Verification items for the finished model (mm, model axes). Give positions to 0.01 mm unless a question says otherwise; leave off trailing zeros. Write each loop counter-clockwise with the first axis right and the second up, starting at its lowest first coordinate (ties: lowest second). Pieces come first, ordered by that corner, then holes. Notation, with made-up numbers: (-1, -10.5) -> (53, -10.5) arc R24 cw to (53, 19.5) -> close; hole circle Ø11 at (-31, 57.5). An arc over 180 degrees is marked (long way). Write item = value, one per line.
from build123d import *

# Parameters (mm, degrees)
SKETCH1_W           = 127
SKETCH1_H           = 76.2
BOSS_EXTRUDE1_DEPTH = 6.35
CUT_EXTRUDE1_REACH  = 8.35
SKETCH2_R           = 1.905


with BuildPart() as part:
    # Sketch1 → Boss-Extrude1 (new body)
    with BuildSketch(Plane.XY):
        with Locations((63.5, -38.1)):
            Rectangle(SKETCH1_W, SKETCH1_H)
    extrude(amount=BOSS_EXTRUDE1_DEPTH)

    # Sketch2 → Cut-Extrude1 (cut, up to next)
    with BuildSketch(Plane.XY.offset(6.35), mode=Mode.PRIVATE) as cut_extrude1_sk1:
        with Locations((82.55, -31.75)):
            Circle(SKETCH2_R)
    cut_extrude1_tool1 = extrude(cut_extrude1_sk1.sketch, amount=-CUT_EXTRUDE1_REACH, mode=Mode.PRIVATE) & part.part
    add(cut_extrude1_tool1.solids().sort_by_distance((82.55, -31.75, 6.35))[0], mode=Mode.SUBTRACT)
    # Sketch2 → Cut-Extrude1 (cut, up to next)
    with BuildSketch(Plane.XY.offset(6.35), mode=Mode.PRIVATE) as cut_extrude1_sk2:
        with Locations((120.65, -31.75)):
            Circle(SKETCH2_R)
    cut_extrude1_tool2 = extrude(cut_extrude1_sk2.sketch, amount=-CUT_EXTRUDE1_REACH, mode=Mode.PRIVATE) & part.part
    add(cut_extrude1_tool2.solids().sort_by_distance((120.65, -31.75, 6.35))[0], mode=Mode.SUBTRACT)
    # Sketch2 → Cut-Extrude1 (cut, up to next)
    with BuildSketch(Plane.XY.offset(6.35), mode=Mode.PRIVATE) as cut_extrude1_sk3:
        with Locations((82.55, -69.85)):
            Circle(SKETCH2_R)
    cut_extrude1_tool3 = extrude(cut_extrude1_sk3.sketch, amount=-CUT_EXTRUDE1_REACH, mode=Mode.PRIVATE) & part.part
    add(cut_extrude1_tool3.solids().sort_by_distance((82.55, -69.85, 6.35))[0], mode=Mode.SUBTRACT)
    # Sketch2 → Cut-Extrude1 (cut, up to next)
    with BuildSketch(Plane.XY.offset(6.35), mode=Mode.PRIVATE) as cut_extrude1_sk4:
        with Locations((120.65, -69.85)):
            Circle(SKETCH2_R)
    cut_extrude1_tool4 = extrude(cut_extrude1_sk4.sketch, amount=-CUT_EXTRUDE1_REACH, mode=Mode.PRIVATE) & part.part
    add(cut_extrude1_tool4.solids().sort_by_distance((120.65, -69.85, 6.35))[0], mode=Mode.SUBTRACT)
    # Sketch2 → Cut-Extrude1 (cut, up to next)
    with BuildSketch(Plane.XY.offset(6.35), mode=Mode.PRIVATE) as cut_extrude1_sk5:
        with Locations((6.35, -50.8)):
            Circle(SKETCH2_R)
    cut_extrude1_tool5 = extrude(cut_extrude1_sk5.sketch, amount=-CUT_EXTRUDE1_REACH, mode=Mode.PRIVATE) & part.part
    add(cut_extrude1_tool5.solids().sort_by_distance((6.35, -50.8, 6.35))[0], mode=Mode.SUBTRACT)


solid = part.part
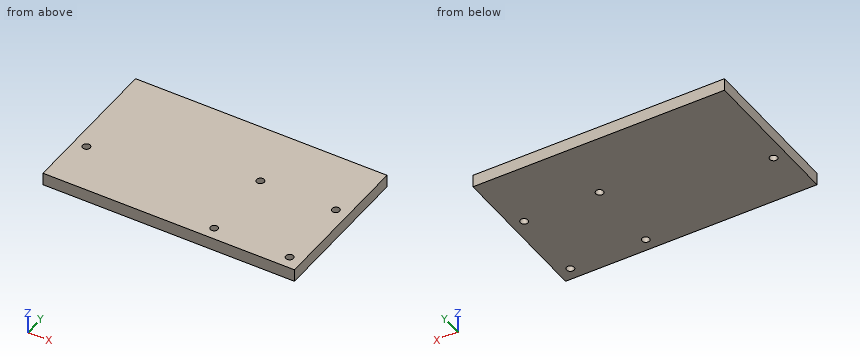
Item 1: Sectioned sample at C-C on y = -31.75. Record the cut outline in (x, z) (3 decimals), then the cut area to 3 significant figures.
Response values:
outline = (0, 0) -> (80.645, 0) -> (80.645, 6.35) -> (0, 6.35) -> close; (84.455, 0) -> (118.745, 0) -> (118.745, 6.35) -> (84.455, 6.35) -> close; (122.555, 0) -> (127, 0) -> (127, 6.35) -> (122.555, 6.35) -> close
area = 758 mm^2
Item 2: Sectioned sample at A-A on y = -50.8. Record the cut outline in (x, z) (3 decimals), then the cut area to 3 significant figures.
Response values:
outline = (0, 0) -> (4.445, 0) -> (4.445, 6.35) -> (0, 6.35) -> close; (8.255, 0) -> (127, 0) -> (127, 6.35) -> (8.255, 6.35) -> close
area = 782 mm^2
Item 3: Material ranges on line 1 (X direction, y = -69.85, z = 1.75) (3 decimals); line 2 (Y direction, x = 82.55, z = 2.25) (3 decimals); line 3 (Y direction, x = 81, z = 4.5), recorded low to high.
Response values:
line_1 = 0 to 80.645, 84.455 to 118.745, 122.555 to 127
line_2 = -76.2 to -71.755, -67.945 to -33.655, -29.845 to 0
line_3 = -76.2 to -70.96, -68.74 to -32.86, -30.64 to 0
Item 4: Sectioned sample at B-B on x = 82.55. Record the cut outline in (y, z) (3 decimals).
Response values:
outline = (-76.2, 0) -> (-71.755, 0) -> (-71.755, 6.35) -> (-76.2, 6.35) -> close; (-67.945, 0) -> (-33.655, 0) -> (-33.655, 6.35) -> (-67.945, 6.35) -> close; (-29.845, 0) -> (0, 0) -> (0, 6.35) -> (-29.845, 6.35) -> close
